Source: CAD feature listing. Evaluate the final solid. Frame: model axes, mm. Face numbers are marked on the shaded views. A direction names the side the tool comes from. Round coordinates to 2 decimals unless told otherwise and drop trailing zeros. Write each loop counter-clockwise with the first axis right and the second up, starting at its lowest first coordinate (ties: lowest second). Pieces come first, ordered by that corner, then holes.
Solid Edge part; units mm, degrees
sketch "Sketch1" plane through (0, 0, 0) normal (1, 0, 0) x (0, 1, 0)
  line L0 (0, 0) -> (0, 35)
  line L1 (0, 35) -> (2, 35)
  line L2 (2, 35) -> (2, 0)
  line L3 (2, 0) -> (0, 0)
extrude "Protrusion1" add sketch "Sketch1" along normal mid plane 68
sketch "Sketch2" plane through (0, 0, 0) normal (1, 0, 0) x (0, 1, 0)
  line L0 (-55, 37) -> (0, 37)
  line L1 (2, 37) -> (0, 37)
  line L2 (2, 37) -> (2, 35)
  line L3 (0, 35) -> (2, 35)
  line L4 (0, 35) -> (-55, 35)
  line L5 (-55, 35) -> (-55, 37)
extrude "ExtrudedProtrusion_2" add sketch "Sketch2" along normal mid plane 125
sketch "Sketch3" plane through (0, -26.5, 37) normal (0, 0, 1) x (1, 0, 0)
  circle A0 centre (-52.3239, -17.6363) radius 2.5
  circle A1 centre (52.3239, -17.6363) radius 2.5
extrude "ExtrudedCutout_1" cut sketch "Sketch3" against normal blind 8.7921
sketch "Sketch4" plane through (0, 0, 17.5) normal (0, -1, 0) x (1, 0, 0)
  circle A0 centre (-22, -11.8558) radius 2.5
  circle A1 centre (22, -11.8558) radius 2.5
extrude "ExtrudedCutout_2" cut sketch "Sketch4" against normal blind 47.6347
sketch "Sketch5" plane through (0, 2, 18.5) normal (0, 1, 0) x (-1, 0, 0)
  line L0 (-36, -18.5) -> (-36, 16.5)
  line L1 (-36, 16.5) -> (-34, 16.5)
  line L2 (-34, 16.5) -> (-34, -18.5)
  line L3 (-34, -18.5) -> (-36, -18.5)
  line L4 (36, 16.5) -> (36, -18.5)
  line L5 (36, -18.5) -> (34, -18.5)
  line L6 (34, -18.5) -> (34, 16.5)
  line L7 (34, 16.5) -> (36, 16.5)
extrude "ExtrudedProtrusion_3" add sketch "Sketch5" against normal up to vertex (2 mm away) and the other way blind 15
fillet "Round_1" radius 5.06 2 edges at (36, 0, 17.5) (-36, 0, 17.5)
fillet "Round_2" radius 2 1 edges at (34, 2, 17.5)
fillet "Round_3" radius 2 1 edges at (-34, 2, 17.5)
fillet "Round_5" radius 2 2 edges at (33.4849, 2, 35) (-33.4849, 2, 35)
fillet "Round_6" radius 10 2 edges at (-62.5, -55, 36) (62.5, -55, 36)
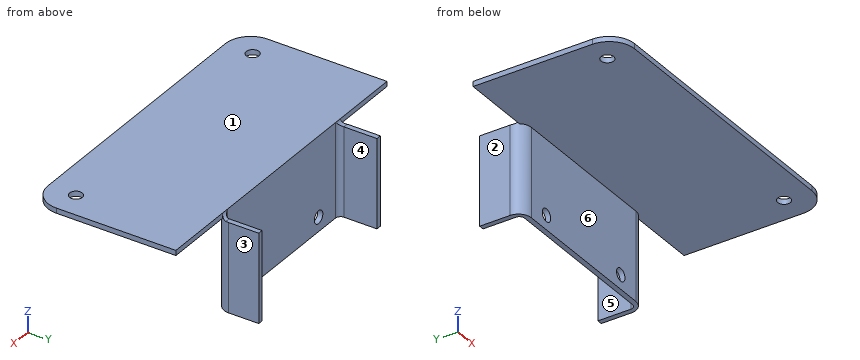
Q1. Set-up query: the marked faces 5 and 6. Return all of +Z, -Z, +X, -X, +Y, -Y with unobstructed straight access to the full face (end or side cutting, diameter ignored); none if empty.
Q2. Line query: line 1 (X direction, y = 10.5, z = 15.5); line 2 (X direction, y = 1, z = 5.5); line 3 (Z direction, x = 22, y = 1.35). Output: solid intervals per line, ascending.
Q3. Pin query (flat end, axial travel): P1, Ø13, axis at y = 12, z = 17, coming from the +X side; P2, Ø4, axis at x = -22, z = 5.64, coming from the -Y side; P3, Ø8, axis at x = -10.5, z = 12.5, coming from the -Y side; P4, Ø8, axis at x = -52.32, y = -44.14, coming from the -Z side. Return the tip coordinate at first contact, or that it passes through.
Q4. Mould query, pull axis X, two halves, no side actions, for the marked faces 1, 2, 3 and 4. Classes: pulls with the +X half, pulls with the -X half, needs draft (parallel to the pull), parting line crosses it, or undercut.
Q5. Section query C-C, the plane y = -13. Output: boundary loops of the cut face in (x, z), and give its area (3 significant figures).
Q6. Section query B-B, the plane z = 32. Output: boundary loops of the cut face in (x, y), and give its area (3 significant figures).
Q7. Section query A-A, the plane x = -22. Output: boundary loops of the cut face in (y, z).
Filled in:
1. face 5: +Z, -Z, +Y
1. face 6: -Z, +X, -X, -Y
2. line 1: x = -36 to -34, 34 to 36
2. line 2: x = -33.96 to -24.5, -19.5 to 19.5, 24.5 to 33.96
2. line 3: z = 0 to 3.14, 8.14 to 37
3. P1: stops at x = 36
3. P2: passes through
3. P3: stops at y = 0
3. P4: stops at z = 35
4. face 1: needs draft
4. face 2: pulls with the -X half
4. face 3: pulls with the +X half
4. face 4: undercut
5. outline: (-62.5, 35) - (62.5, 35) - (62.5, 37) - (-62.5, 37) - close
5. area: 250 mm2
6. outline: (-36, 5.06) arc R5.06 ccw to (-30.94, 0) - (30.94, 0) arc R5.06 ccw to (36, 5.06) - (36, 17) - (34, 17) - (34, 4) arc R2 cw to (32, 2) - (-32, 2) arc R2 cw to (-34, 4) - (-34, 17) - (-36, 17) - close
6. area: 195 mm2
7. outline: (-55, 35) - (0, 35) - (0, 8.14) - (2, 8.14) - (2, 37) - (-55, 37) - close; (0, 0) - (2, 0) - (2, 3.14) - (0, 3.14) - close
